Read the model definition and answer for the solid it produces. Units are mm, in the model's axes. A direction names the side the tool comes from. Coordinates: 2 decimals unless noted, no trailing zeros. Loops run counter-clockwise (first coordinate to the right, second up) from the corner with the lowest first, then second, coordinate; pieces in that order, holes last. Notation, with made-up numbers: (-38, 14) - (-8, 14) arc R22 ccw to (-8, 37) - close; hole circle Ø2 at (-1.5, 84). An arc over 180 degrees is marked (long way). Use one line per item in the form item = value.
from build123d import *

# Parameters (mm, degrees)
SKETCH1_R                = 6
BOSS_EXTRUDE1_DEPTH      = 100
SKETCH5_R                = 3.05
CUT_EXTRUDE1_DEPTH       = 2.2
CHAMFER1_SIZE            = 0.2
CUT_EXTRUDE2_DEPTH       = 201.179919073
CUT_EXTRUDE4_DEPTH       = 10
CHAMFER3_SIZE            = 0.54
CHAMFER3_OF_MIRROR3_SIZE = 0.54


with BuildPart() as part:
    # Sketch1 → Boss-Extrude1 (new, symmetric)
    with BuildSketch(Plane.XY):
        Circle(SKETCH1_R)
    extrude(amount=BOSS_EXTRUDE1_DEPTH, both=True)

    # Sketch4 → Hole1 (revolve, cut)
    with BuildSketch(Plane(origin=(0, 0, 100), x_dir=(0, -1, 0), z_dir=(1, 0, 0))):
        Polygon((0, 0), (0, 13.85), (1.85, 12), (1.85, 0), align=None)
    hole1 = revolve(axis=Axis((0, 0, 104.244199587), (0, 0, -1)), mode=Mode.SUBTRACT)

    # Sketch5 → Cut-Extrude1 (cut)
    with BuildSketch(Plane.XY.offset(100)):
        Circle(SKETCH5_R)
    cut_extrude1 = extrude(amount=-CUT_EXTRUDE1_DEPTH, mode=Mode.SUBTRACT)

    # Mirror2: Hole1, Cut-Extrude1 across plane
    add(hole1.mirror(Plane.XY), mode=Mode.SUBTRACT)
    add(cut_extrude1.mirror(Plane.XY), mode=Mode.SUBTRACT)

    # Chamfer1
    chamfer1_edges = [part.edges().sort_by_distance(p)[0] for p in [
        (-3.05, 0, 100),
        (0, 1.85, 97.8),
        (-3.05, 0, -100),
        (0, 1.85, -97.8),
    ]]
    chamfer(chamfer1_edges, length=CHAMFER1_SIZE)

    # Sketch6 → Cut-Extrude2 (cut, through all)
    with BuildSketch(Plane.XY.offset(100)):
        with BuildLine():
            Line((2.047046653, -5.64), (-2.047046653, -5.64))
            ThreePointArc((-2.047046653, -5.64), (0, -6), (2.047046653, -5.64))
        make_face()
    extrude(amount=-CUT_EXTRUDE2_DEPTH, mode=Mode.SUBTRACT)

    # Sketch9 → Cut-Extrude4 (cut)
    with BuildSketch(Plane.XY.offset(100)):
        with BuildLine():
            Line((-5.5, -2.397915762), (-5.5, 2.397915762))
            ThreePointArc((-5.5, 2.397915762), (-6, 0), (-5.5, -2.397915762))
        make_face()
        with BuildLine():
            Line((5.5, -2.397915762), (5.5, 2.397915762))
            ThreePointArc((5.5, 2.397915762), (6, 0), (5.5, -2.397915762))
        make_face()
    cut_extrude4 = extrude(amount=-CUT_EXTRUDE4_DEPTH, mode=Mode.SUBTRACT)

    # Chamfer3
    # the kernel refuses this chamfer: 0.54 mm, written as the material it adds along each edge
    with BuildSketch(Plane(origin=(5.5, -3.786624575, 90), x_dir=(-0.027495876610584932, 0, 0.9996219169112968), z_dir=(0, 1, 0))) as chamfer3_piece_1_section:
        Polygon((CHAMFER3_SIZE * 0.999621916911, CHAMFER3_SIZE * 0.0274958766106), (-CHAMFER3_SIZE * 0.0274958766106, CHAMFER3_SIZE * 0.999621916911), (0, 0), align=None)
    chamfer3_piece_1 = extrude(amount=7.57324915, mode=Mode.PRIVATE)
    chamfer3_piece_1 = chamfer3_piece_1 & Plane(origin=(0, 0, 90.196712304), x_dir=(1, 0, 0), z_dir=(0, 0, 1)) * Cylinder(6, 18, mode=Mode.PRIVATE)
    add(chamfer3_piece_1)
    with BuildSketch(Plane(origin=(-5.5, -3.786624575, 90), x_dir=(0.027495876610584932, 0, 0.9996219169112968), z_dir=(0, 1, 0))) as chamfer3_piece_2_section:
        Polygon((CHAMFER3_SIZE * 0.999621916911, -CHAMFER3_SIZE * 0.0274958766106), (-CHAMFER3_SIZE * 0.0274958766106, -CHAMFER3_SIZE * 0.999621916911), (0, 0), align=None)
    chamfer3_piece_2 = extrude(amount=7.57324915, mode=Mode.PRIVATE)
    chamfer3_piece_2 = chamfer3_piece_2 & Plane(origin=(0, 0, 90.196712302), x_dir=(1, 0, 0), z_dir=(0, 0, 1)) * Cylinder(6, 18, mode=Mode.PRIVATE)
    add(chamfer3_piece_2)

    # Mirror3: Cut-Extrude4 across plane
    add(cut_extrude4.mirror(Plane.XY), mode=Mode.SUBTRACT)

    # Chamfer3 of Mirror3
    # the kernel refuses this chamfer: 0.54 mm, written as the material it adds along each edge
    with BuildSketch(Plane(origin=(5.5, -3.786624575, -90), x_dir=(-0.027495876610584932, 0, -0.9996219169112968), z_dir=(0, 1, 0))) as chamfer3_of_mirror3_piece_1_section:
        Polygon((CHAMFER3_OF_MIRROR3_SIZE * 0.999621916911, -CHAMFER3_OF_MIRROR3_SIZE * 0.0274958766106), (-CHAMFER3_OF_MIRROR3_SIZE * 0.0274958766106, -CHAMFER3_OF_MIRROR3_SIZE * 0.999621916911), (0, 0), align=None)
    chamfer3_of_mirror3_piece_1 = extrude(amount=7.57324915, mode=Mode.PRIVATE)
    chamfer3_of_mirror3_piece_1 = chamfer3_of_mirror3_piece_1 & Plane(origin=(0, 0, -90.196712304), x_dir=(1, 0, 0), z_dir=(0, 0, 1)) * Cylinder(6, 18, mode=Mode.PRIVATE)
    add(chamfer3_of_mirror3_piece_1)
    with BuildSketch(Plane(origin=(-5.5, -3.786624575, -90), x_dir=(0.027495876610584932, 0, -0.9996219169112968), z_dir=(0, 1, 0))) as chamfer3_of_mirror3_piece_2_section:
        Polygon((CHAMFER3_OF_MIRROR3_SIZE * 0.999621916911, CHAMFER3_OF_MIRROR3_SIZE * 0.0274958766106), (-CHAMFER3_OF_MIRROR3_SIZE * 0.0274958766106, CHAMFER3_OF_MIRROR3_SIZE * 0.999621916911), (0, 0), align=None)
    chamfer3_of_mirror3_piece_2 = extrude(amount=7.57324915, mode=Mode.PRIVATE)
    chamfer3_of_mirror3_piece_2 = chamfer3_of_mirror3_piece_2 & Plane(origin=(0, 0, -90.196712302), x_dir=(1, 0, 0), z_dir=(0, 0, 1)) * Cylinder(6, 18, mode=Mode.PRIVATE)
    add(chamfer3_of_mirror3_piece_2)


solid = part.part
Item 1: For a pull along X with two mould halves and no side action, classify faces 4 (the cylindrical face through (1.806, 0.401, 92.867)), 5 (the flat face through (5.5, 0, -95)), 6 (the flat face through (-3, -2, -100)), 7 (the flat face through (-5.5, 0, -95)) as +X half, -X half, draft (parallel to the pull), parting line (faces both ways), or undercut.
Results below:
face_4 = undercut
face_5 = +X half
face_6 = draft
face_7 = -X half
Item 2: Each of these flat-tipped pins is pushed along its axis until it touches: P1, Ø5, axis at x = -0.5, y = -0.5, coming from the -Z side; P2, Ø3, axis at x = 0, y = 0, coming from the -Z side; P3, Ø1, axis at x = -3, z = 80, coming from the +Y side. Where does it stop, or does it pass through?
Results below:
P1 = -99.96
P2 = -87.65
P3 = 5.45
Item 3: Which of the six approach directions +Z, -Z, +X, -X, +Y, -Y give full straight-line access (tool end or side, diameter ignored) to faces 1 (the flat face through (-5.5, 0, 95)), 2 (the cylindrical face through (-3.047, 0.134, 98.814)), 3 (the cylindrical face through (1.806, 0.401, -92.867))?
Results below:
face_1 = +Z, -X, +Y, -Y
face_2 = +Z
face_3 = -Z
Item 4: The part is cut by section A-A on z = -66. Give the vertices of the cut face in (x, y).
Results below:
outline = (-2.05, -5.64) - (2.05, -5.64) arc R6 ccw (long way) to start
Item 5: Find the intervals of material crossed by L1, parallel to Y at x = 0, z = 90.75; L2, parallel to X at y = -0.5, z = 2; L3, parallel to Z at x = -2.5, y = 0, in increasing order.
Results below:
L1 = -5.64 to -1.85, 1.85 to 6
L2 = -5.98 to 5.98
L3 = -97.8 to 97.8
